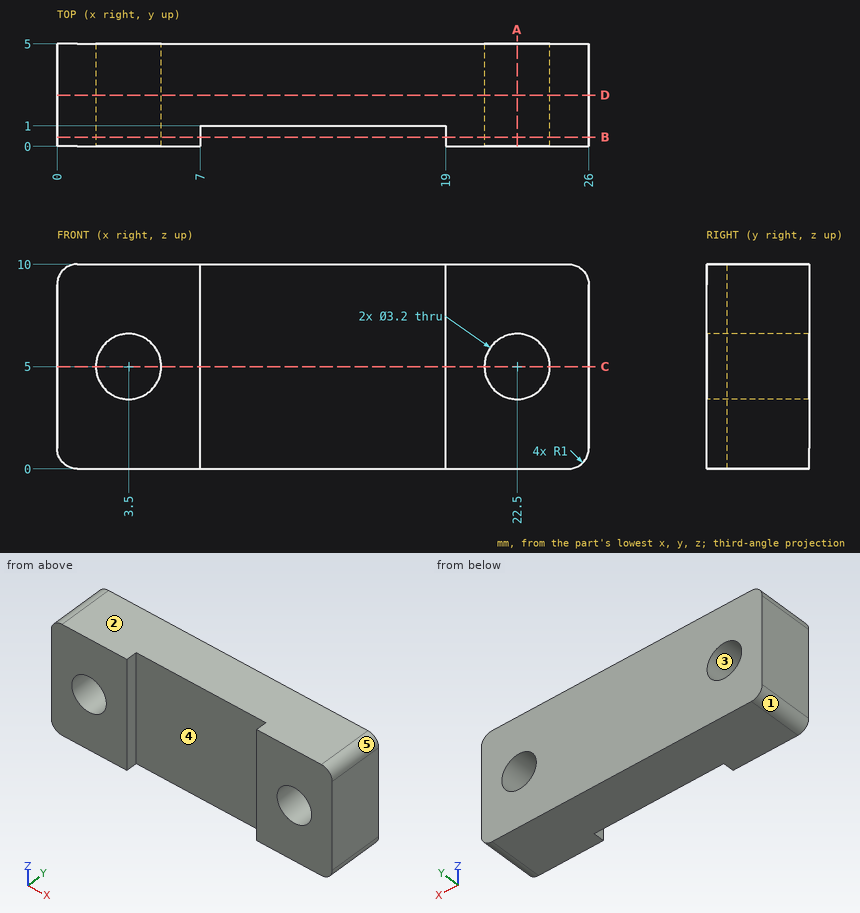
For this review, use the dimensioned drawing (mm, ordinates from the lowest corner) and the shaded views. A direction names the side the tool comes from. Give positions to 0.01 mm unless a question says otherwise; leave off trailing zeros. Write each loop counter-clockwise with the first axis right and the second up, starting at its lowest first coordinate (ties: lowest second). Pieces come first, ordered by that corner, then holes. Notation, with made-up numbers: M 46.25,57 L 76.25,57 A20 ccw 76.25,63 Z; hole C -30.75,84.25 d3. An arc over 180 degrees is marked long. Answer as a JSON object with one key per item and string values. Group by question number.
1) We need section C-C (z = 5). Give the boundary of the cut face in (x, y).
2) We need section D-D (y = 2.5). Give the boundary of the cut face in (x, z).
3) We need section B-B (y = 0.45). Give the boundary of the cut face in (x, z), and give its area (3 significant figures).
4) For line 1 along Z through (x, y) = (22.5, 2.45); line 2 along X through (y, z) = (0.9, 8.25); line 3 along X through (y, z) = (1.75, 5.5), list the stretches that pass through material, from the lowest coordinate up.
5) Mouldability with a two-part tool opening along X and no side actions: class the marked faces 1, 2 and 3 as released by +X, released by -X, zero draft, split by the parting line, or undercut.
6) Clearance check with a flat-ended pin moving along its axis: pin 1 Ø5 at (x, z) = (11, 7) entering from -Y. State where the tip first meets the part, or that it passes through.
7) Tool access review of the marked faces 4 and 5: name each direction out of +Z, -Z, +X, -X, +Y, -Y from which nothing blocks a thin tool from reaching the whole face with its end or side.
8) We need section A-A (x = 22.5). Give the boundary of the cut face in (y, z).
Answer key:
{
 "1": {"outline": "M 0,0 L 1.9,0 L 1.9,5 L 0,5 Z; M 5.1,0 L 7,0 L 7,1 L 19,1 L 19,0 L 20.9,0 L 20.9,5 L 5.1,5 Z; M 24.1,0 L 26,0 L 26,5 L 24.1,5 Z"},
 "2": {"outline": "M 0,1 A1 ccw 1,0 L 25,0 A1 ccw 26,1 L 26,9 A1 ccw 25,10 L 1,10 A1 ccw 0,9 Z; hole C 3.5,5 d3.2; hole C 22.5,5 d3.2"},
 "3": {"outline": "M 0,1 A1 ccw 1,0 L 7,0 L 7,10 L 1,10 A1 ccw 0,9 Z; M 19,0 L 25,0 A1 ccw 26,1 L 26,9 A1 ccw 25,10 L 19,10 Z; hole C 3.5,5 d3.2; hole C 22.5,5 d3.2", "area": "123 mm²"},
 "4": {"line 1": "z = 0 to 3.4, 6.6 to 10", "line 2": "x = 0 to 7, 19 to 26", "line 3": "x = 0 to 1.98, 5.02 to 20.98, 24.02 to 26"},
 "5": {"face 1": "released by -X", "face 2": "zero draft", "face 3": "undercut"},
 "6": {"pin 1": "stops at y = 1"},
 "7": {"face 4": "+Z, -Z, -Y", "face 5": "+Z, +X, +Y, -Y"},
 "8": {"outline": "M 0,0 L 5,0 L 5,3.4 L 0,3.4 Z; M 0,6.6 L 5,6.6 L 5,10 L 0,10 Z"}
}
